CAD build for the part. Positions are in the model's coordinates, mm. Face numbers are marked on the shaded views. A direction names the side the tool comes from. Coordinates: 2 decimals unless noted, no trailing zeros. Order: outer loops, then holes, each group sorted by start corner. A loop starts at its lowest first (then second) coordinate and runs counter-clockwise, first axis right, second up. Notation, with made-up numbers: (-16.75, -18.75) - (-2.75, -18.75) arc R19 ccw to (-2.75, 5.25) - close; hole circle Ø2 at (68, 82). An arc over 180 degrees is marked (long way). Use one line per item in the form item = value.
```python
from build123d import *

# Parameters (mm, degrees)
SKETCH1_R                                           = 34.925
BOSS_EXTRUDE1_DEPTH                                 = 12.7
CBORE_FOR_10_BINDING_HEAD_MACHINE_SCREW_D           = 5.08
CBORE_FOR_10_BINDING_HEAD_MACHINE_SCREW_CBORE_D     = 11.1125
CBORE_FOR_10_BINDING_HEAD_MACHINE_SCREW_CBORE_DEPTH = 6.35


with BuildPart() as part:
    # Sketch1 → Boss-Extrude1 (new body)
    with BuildSketch(Plane.XY):
        Circle(SKETCH1_R)
    extrude(amount=BOSS_EXTRUDE1_DEPTH)

    # CBORE for #10 Binding Head Machine Screw1 (through all)
    with Locations(Plane(origin=(0, 0, 0), x_dir=(1, 0, 0), z_dir=(0, 0, -1))):
        with Locations((0, -11.641666667), (0, 11.641666667)):
            CounterBoreHole(CBORE_FOR_10_BINDING_HEAD_MACHINE_SCREW_D / 2, CBORE_FOR_10_BINDING_HEAD_MACHINE_SCREW_CBORE_D / 2, CBORE_FOR_10_BINDING_HEAD_MACHINE_SCREW_CBORE_DEPTH)


solid = part.part
```
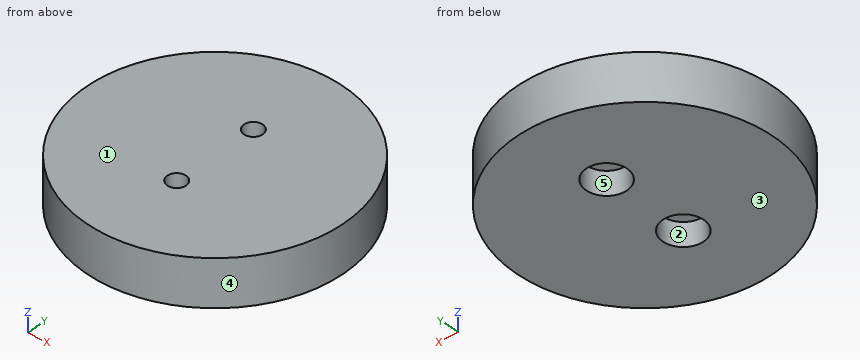
Item 1: Cut at B-B, the plane y = -15. Write the cut outline in (x, z), plus the area to 3 significant figures.
Derived:
outline = (-31.54, 0) - (-4.43, 0) - (-4.43, 6.35) - (4.43, 6.35) - (4.43, 0) - (31.54, 0) - (31.54, 12.7) - (-31.54, 12.7) - close
area = 745 mm²
Item 2: Cut at C-C, the plane z = 3.5. State how many separate pieces and enclosed holes the cut face has, plus the area to 3 significant figures.
Derived:
separate_pieces = 1
enclosed_holes = 2
area = 3,640 mm²
Item 3: Drill centre lines: line 1 (Y direction, x = 0, z = 1.75) (3 decimals); line 2 (Y direction, x = 0, z = 11.5) (3 decimals); line 3 (X direction, y = 0.5, z = 7.75). Where is each one in solid material? Low to high. Write a range as [from, to].
Derived:
line_1 = [-34.925, -17.198], [-6.085, 6.085], [17.198, 34.925]
line_2 = [-34.925, -14.182], [-9.102, 9.102], [14.182, 34.925]
line_3 = [-34.92, 34.92]
Item 4: 3-axis set-ups, long thin cutter, end or side, ignore diameter. For the marked faces 1 and 2: which of +Z, -Z, +X, -X, +Y, -Y reach the whole face in a straight line?
Derived:
face_1 = +Z, +X, -X, +Y, -Y
face_2 = -Z
Item 5: Two-plate mould, pull along Y, no slides. Class the marked faces 3, 4 and 5: +Y half, -Y half, draft (parallel to the pull), parting line (faces both ways), or undercut.
Derived:
face_3 = draft
face_4 = parting line
face_5 = undercut
Item 6: Drop flat-ended pins along their axis: pin 1 (5 mm diameter, centred on y = -27.5, z = 5.5, fed in from +X); pin 2 (1.5 mm diameter, centred on x = 2.5, z = 5, fed in from -Y); pin 3 (9 mm diameter, centred on x = -1, y = -14.5, fed in from -Z); pin 4 (2 mm diameter, centred on x = 7.5, z = 11, fed in from -Y). Give the stop position or say it passes through.
Derived:
pin_1 = 24.39
pin_2 = -34.88
pin_3 = 0
pin_4 = -34.31
Item 7: Cut at A-A, the plane x = 0. Write the cut outline in (y, z) (3 decimals).
Derived:
outline = (-34.925, 0) - (-17.198, 0) - (-17.198, 6.35) - (-14.182, 6.35) - (-14.182, 12.7) - (-34.925, 12.7) - close; (-9.102, 6.35) - (-6.085, 6.35) - (-6.085, 0) - (6.085, 0) - (6.085, 6.35) - (9.102, 6.35) - (9.102, 12.7) - (-9.102, 12.7) - close; (14.182, 6.35) - (17.198, 6.35) - (17.198, 0) - (34.925, 0) - (34.925, 12.7) - (14.182, 12.7) - close
Item 8: Cut at D-D, the plane x = 26. Write the cut outline in (y, z).
Derived:
outline = (-23.32, 0) - (23.32, 0) - (23.32, 12.7) - (-23.32, 12.7) - close
